Part model, mm, in its own coordinate system. A direction names the side the tool comes from. Coordinates: 2 decimals unless noted, no trailing zeros. Order: outer loops, then holes, each group sorted by start corner. A loop starts at its lowest first (then second) coordinate and runs counter-clockwise, first axis right, second up.
from build123d import *

# Parameters (mm, degrees)
SKETCH1_W               = 127
SKETCH1_H               = 28.575
BOSS_EXTRUDE1_DEPTH     = 25.4
CUT_EXTRUDE3_DEPTH      = 45.72
CUT_EXTRUDE3_DEPTH_BACK = 55.88
FILLET1_R               = 12.7
SKETCH6_R               = 6.35
CUT_EXTRUDE5_DEPTH      = 31.75
CUT_EXTRUDE6_DEPTH      = 31.75
SKETCH8_W               = 88.9
SKETCH8_H               = 19.05
CUT_EXTRUDE7_DEPTH      = 17.4625
FILLET2_R               = 7.62
SKETCH10_R              = 4.7625
CUT_EXTRUDE8_DEPTH      = 42.8625
SKETCH11_W              = 6.189214409
SKETCH11_H              = 19.05
SKETCH11_W_2            = 6.35
CUT_EXTRUDE10_DEPTH     = 8.0645
FILLET3_R               = 1.524
FILLET4_R               = 2.54


with BuildPart() as part:
    # Sketch1 → Boss-Extrude1 (new body)
    with BuildSketch(Plane(origin=(0, 0, 0), x_dir=(1, 0, 0), z_dir=(0, 1, 0))):
        with Locations((63.5, 14.2875)):
            Rectangle(SKETCH1_W, SKETCH1_H)
    extrude(amount=BOSS_EXTRUDE1_DEPTH)

    # Sketch5 → Cut-Extrude3 (cut, two sides: drawn at the far end of the back side and taken through both)
    with BuildSketch(Plane(origin=(0, 25.4, 0), x_dir=(1, 0, 0), z_dir=(0, 1, 0)).offset(-CUT_EXTRUDE3_DEPTH_BACK)):
        with BuildLine():
            Line((19.05, 0), (50.8, 0))
            ThreePointArc((50.8, 0), (34.925, 7.816775665), (19.05, 0))
        make_face()
    extrude(amount=CUT_EXTRUDE3_DEPTH + CUT_EXTRUDE3_DEPTH_BACK, mode=Mode.SUBTRACT)

    # Fillet1
    fillet1_edges = [part.edges().sort_by_distance(p)[0] for p in [
        (0, 12.7, -28.575),
        (0, 12.7, 0),
    ]]
    fillet(fillet1_edges, radius=FILLET1_R)

    # Sketch6 → Cut-Extrude5 (cut)
    with BuildSketch(Plane(origin=(0, 25.4, 0), x_dir=(1, 0, 0), z_dir=(0, 1, 0))):
        with Locations(Location((12.7, 12.7, 0), (0, 0, 270))):
            Circle(SKETCH6_R)
    extrude(amount=-CUT_EXTRUDE5_DEPTH, mode=Mode.SUBTRACT)

    # Sketch7 → Cut-Extrude6 (cut)
    with BuildSketch(Plane(origin=(0, 25.4, 0), x_dir=(1, 0, 0), z_dir=(0, 1, 0))):
        with BuildLine():
            Line((11.913860826, 25.375645356), (63.5, 28.575))
            Line((63.5, 28.575), (12.7, 28.575))
            ThreePointArc((12.7, 28.575), (3.719743879, 24.855256121), (0, 15.875))
            Line((0, 15.875), (0, 12.7))
            ThreePointArc((0, 12.7), (3.445974727, 21.397874237), (11.913860826, 25.375645356))
        make_face()
    extrude(amount=-CUT_EXTRUDE6_DEPTH, mode=Mode.SUBTRACT)

    # Sketch8 → Cut-Extrude7 (cut)
    with BuildSketch(Plane.XY):
        with Locations((79.375, 12.7)):
            Rectangle(SKETCH8_W, SKETCH8_H)
    extrude(amount=-CUT_EXTRUDE7_DEPTH, mode=Mode.SUBTRACT)

    # Fillet2
    # the kernel refuses this fillet: 7.62 mm, written as the material it takes off along each edge
    with BuildSketch(Plane(origin=(127, -19.05, 0), x_dir=(-1, 0, 0), z_dir=(0, 1, 0))) as fillet2_piece_1:
        with BuildLine():
            CenterArc((FILLET2_R, -FILLET2_R), FILLET2_R, 90, 90)
            Line((0, -FILLET2_R), (0, 0))
            Line((0, 0), (FILLET2_R, 0))
        make_face()
    extrude(amount=63.5, mode=Mode.SUBTRACT)

    # Sketch10 → Cut-Extrude8 (cut)
    with BuildSketch(Plane.XZ):
        with Locations(Location((118.820602805, -7.62, 0), (0, 0, 270))):
            Circle(SKETCH10_R)
    extrude(amount=-CUT_EXTRUDE8_DEPTH, mode=Mode.SUBTRACT)

    # Sketch11 → Cut-Extrude10 (cut)
    with BuildSketch(Plane(origin=(127, 0, 0), x_dir=(0, 0, -1), z_dir=(1, 0, 0))):
        with Locations((4.525392796, 12.7)):
            Rectangle(SKETCH11_W, SKETCH11_H)
        with Locations((10.795, 12.7)):
            Rectangle(SKETCH11_W_2, SKETCH11_H)
    extrude(amount=-CUT_EXTRUDE10_DEPTH, mode=Mode.SUBTRACT)

    # Fillet3
    fillet3_edges = [part.edges().sort_by_distance(p)[0] for p in [
        (123.825, 12.7, -13.97),
        (127, 12.7, -13.97),
        (123.825, 12.7, -17.4625),
    ]]
    fillet(fillet3_edges, radius=FILLET3_R)

    # Fillet4
    fillet4_edges = [part.edges().sort_by_distance(p)[0] for p in [
        (127, 12.7, -28.575),
    ]]
    fillet(fillet4_edges, radius=FILLET4_R)


solid = part.part
Q1. Wall check: line 1 along Y through (x, z) = (113.5, -5) (3 decimals); line 2 along X through (y, z) = (14.5, -12.25) (3 decimals); line 3 along Z through (x, y) = (102, 13.25) (1 decimal). Give the ranges that are in metal, low to high.
Results list:
line 1: y = 0 to 3.175, 22.225 to 25.4
line 2: x = 0.008 to 6.366, 19.034 to 34.925
line 3: z = -28.6 to -17.5
Q2. Which spindle directions (+Z, -Z, +X, -X, +Y, -Y) get a long thin tool onto all of the face, cutting with end or side? Do faces 4 (the face through (82, 3.175, -9)), 5 (the face through (85, 24, 0)). Say none if no direction does.
Results list:
face 4: +Z
face 5: +Z, +X, -X, +Y, -Y
Q3. Cut at B-B on x = 80. Write the cut outline in (y, z) (1 decimal).
Results list:
outline: (0, -28.6) - (25.4, -28.6) - (25.4, 0) - (22.2, 0) - (22.2, -17.5) - (3.2, -17.5) - (3.2, 0) - (0, 0) - close
Q4. Mould opens along X. For faces 1 (the face through (124.709, 23.79, -2.173)), 2 (the face through (63, 0, -14)), 3 (the face through (78, 13, -17.462)) say: pulls with the +X half, pulls with the -X half, needs draft (parallel to the pull), parting line crosses it, or undercut.
Results list:
face 1: pulls with the +X half
face 2: needs draft
face 3: undercut
Q5. Cut at D-D on z = -20.5. Write the cut outline in (x, y).
Results list:
outline: (2.68, 0) - (127, 0) - (127, 25.4) - (2.68, 25.4) - close
Q6. Pin check, flat tips, straight feed: pin 1 Ø12 at (x, y) = (21, 10.5) entering from +Z; pin 2 Ø3 at (x, y) = (109.5, 5.5) entering from +Z; pin 3 Ø4 at (x, y) = (58.5, 9.5) entering from -Z; pin 4 Ø6 at (x, y) = (58.5, 22.5) entering from -Z. Stop position of each tip, or through.
Results list:
pin 1: stops at z = 0
pin 2: stops at z = -17.46
pin 3: stops at z = -28.39
pin 4: stops at z = -28.45
Q7. Cut at C-C on x = 10.5. Write the cut outline in (y, z), and give its area (3 significant figures).
Results list:
outline: (0, -25.21) - (25.4, -25.21) - (25.4, -18.66) - (0, -18.66) - close; (0, -6.74) - (25.4, -6.74) - (25.4, -0.19) - (0, -0.19) - close
area: 333 mm2
